Geometry: final body of the model. Coordinates: model frame, mm. Give positions to 0.01 mm unless a question says otherwise; leave off trailing zeros. Loops run counter-clockwise (first coordinate to the right, second up) from the corner with the lowest first, then second, coordinate; pieces in that order, holes last.
```python
from build123d import *

# Parameters (mm, degrees)
SKETCH5_R           = 48.26
BOSS_EXTRUDE1_DEPTH = 8.89
FILLET1_R           = 25.4
SKETCH9_R           = 2.5527
CUT_EXTRUDE1_DEPTH  = 12.7
FILLET3_R           = 12.7
FILLET4_R           = 12.7
FILLET5_R           = 5.08


with BuildPart() as part:
    # Sketch5 → Boss-Extrude1 (new body)
    with BuildSketch(Plane(origin=(0, 0, 0), x_dir=(1, 0, 0), z_dir=(0, 1, 0))):
        with BuildLine():
            ThreePointArc((-215.9, -46.097790831), (-267.470384182, -127.877406649), (-171.45, -139.168815315))
            Line((-171.45, -139.168815315), (-171.45, -167.709773326))
            Line((-171.45, -167.709773326), (-200.949318136, -200.960227902))
            Line((-200.949318136, -200.960227902), (-177.198993439, -222.031169428))
            Line((-177.198993439, -222.031169428), (-149.225, -190.5))
            Line((-149.225, -190.5), (-127, -190.5))
            Line((-127, -190.5), (-127, 190.5))
            Line((-127, 190.5), (-149.225, 190.5))
            Line((-149.225, 190.5), (-177.198993439, 222.031169428))
            Line((-177.198993439, 222.031169428), (-200.949318136, 200.960227902))
            Line((-200.949318136, 200.960227902), (-171.45, 167.709773326))
            Line((-171.45, 167.709773326), (-171.45, 123.173233653))
            ThreePointArc((-171.45, 123.173233653), (-267.470384182, 111.881824988), (-215.9, 30.102209169))
            Line((-215.9, 30.102209169), (-215.9, -46.097790831))
        make_face()
        with Locations(Location((-215.9, -103.247790831, 0), (0, 0, 270))):
            Circle(SKETCH5_R, mode=Mode.SUBTRACT)
        with Locations(Location((-215.9, 87.252209169, 0), (0, 0, 270))):
            Circle(SKETCH5_R, mode=Mode.SUBTRACT)
    extrude(amount=-BOSS_EXTRUDE1_DEPTH)

    # Fillet1
    # the kernel refuses this fillet: 25.4 mm, written as the material it adds along each edge
    with BuildSketch(Plane(origin=(-171.45, 0, -123.173233653), x_dir=(0, 0, -1), z_dir=(0, -1, 0))) as fillet1_piece_1:
        with BuildLine():
            CenterArc((44.400828084, -25.4), FILLET1_R, 90, 103.342363797)
            Line((19.686411909, -31.261538462), (19.192123586, -31.378769231))
            ThreePointArc((19.192123586, -31.378769231), (12.009069237, -14.266854375), (-0.319297995, -0.395111111))
            Line((-0.319297995, -0.395111111), (0, 0.508))
            Line((0, 0.508), (44.400828084, 0.508))
            Line((44.400828084, 0.508), (44.400828084, 0))
        make_face()
    extrude(amount=8.89)
    with BuildSketch(Plane(origin=(-171.45, 0, 139.168815315), x_dir=(-0.8303696180979097, 0, 0.557212973054228), z_dir=(0, -1, 0))) as fillet1_piece_2:
        with BuildLine():
            CenterArc((41.297101209, -24.264819571), FILLET1_R, 107.194284187, 71.530497093)
            Line((15.903392067, -23.699544404), (15.395517884, -23.6882389))
            ThreePointArc((15.395517884, -23.6882389), (7.529868268, -12.132836392), (-0.421827766, -0.28306419))
            Line((-0.421827766, -0.28306419), (0.150171277, 0.485296391))
            ThreePointArc((0.150171277, 0.485296391), (16.894268676, -2.046155965), (33.638366076, 0.485296391))
            Line((33.638366076, 0.485296391), (33.788537353, 0))
        make_face()
    extrude(amount=8.89)

    # Sketch9 → Cut-Extrude1 (cut)
    with BuildSketch(Plane(origin=(0, 0, 0), x_dir=(1, 0, 0), z_dir=(0, 1, 0))):
        Polygon((-181.61, 8.105163913), (-181.61, 22.76986075), (-194.31, 30.102209169), (-207.01, 22.76986075), (-207.01, 8.105163913), (-194.31, 0.772815494), align=None)
        Polygon((-175.26, -46.887449227), (-175.26, -32.22275239), (-187.96, -24.890403971), (-200.66, -32.22275239), (-200.66, -46.887449227), (-187.96, -54.219797646), align=None)
        Polygon((-175.26, -24.890403971), (-162.56, -17.558055552), (-162.56, -2.893358715), (-175.26, 4.438989704), (-187.96, -2.893358715), (-187.96, -17.558055552), align=None)
        Polygon((-194.31, -6.559532924), (-203.345054514, -1.343141768), (-203.345054514, -26.440620918), (-194.31, -21.224229762), align=None)
        Polygon((-162.56, 33.768383379), (-162.56, 4.438989704), (-175.26, 11.771338122), (-175.26, 26.43603496), align=None)
        Polygon((-162.56, -24.890403971), (-162.56, -46.887449227), (-168.91, -43.221275018), (-168.91, -28.55657818), align=None)
        with Locations(Location((-183.436118723, -153.432579675, 0), (0, 0, 270))):
            Circle(SKETCH9_R)
        with Locations(Location((-138.1125, 183.418546383, 0), (0, 0, 270))):
            Circle(SKETCH9_R)
        with Locations(Location((-138.1125, -184.15, 0), (0, 0, 270))):
            Circle(SKETCH9_R)
        with Locations(Location((-166.939936911, 153.157179019, 0), (0, 0, 270))):
            Circle(SKETCH9_R)
        with Locations(Location((-209.55, -1.647790831, 0), (0, 0, 270))):
            Circle(SKETCH9_R)
        with Locations(Location((-209.55, -33.397790831, 0), (0, 0, 270))):
            Circle(SKETCH9_R)
        with Locations(Location((-209.55, 30.102209169, 0), (0, 0, 270))):
            Circle(SKETCH9_R)
    extrude(amount=-CUT_EXTRUDE1_DEPTH, mode=Mode.SUBTRACT)

    # Fillet3
    fillet3_edges = [part.edges().sort_by_distance(p)[0] for p in [
        (-149.225, -4.445, -190.5),
        (-171.45, -4.445, -167.709773326),
        (-171.45, -4.445, 167.709773326),
        (-149.225, -4.445, 190.5),
    ]]
    fillet(fillet3_edges, radius=FILLET3_R)

    # Fillet4
    fillet4_edges = [part.edges().sort_by_distance(p)[0] for p in [
        (-215.9, -4.445, 46.097790831),
        (-215.9, -4.445, -30.102209169),
    ]]
    fillet(fillet4_edges, radius=FILLET4_R)

    # Fillet5
    fillet5_edges = [part.edges().sort_by_distance(p)[0] for p in [
        (-200.949318136, -4.445, -200.960227902),
        (-177.198993439, -4.445, -222.031169428),
    ]]
    fillet(fillet5_edges, radius=FILLET5_R)


solid = part.part
```
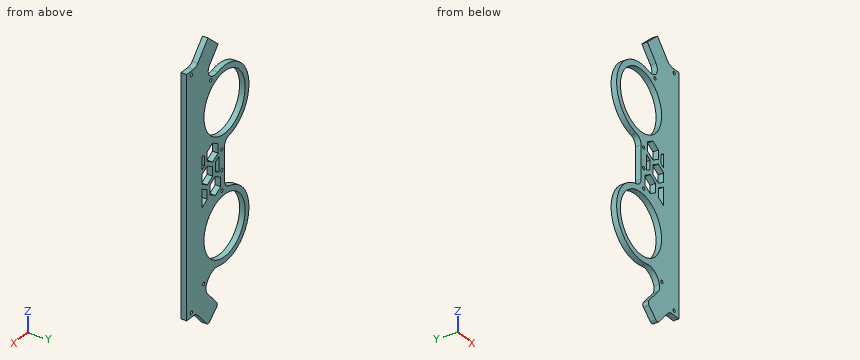
Q1. Pin query (flat end, axial travel): pin 1 Ø4 at (x, z) = (-209.55, 33.4) entering from +Y; pin 2 Ø2.5 at (y, z) = (-6, 38.5) entering from -X; pin 3 Ø2.5 at (x, y) = (-133, -6) entering from +Z; pin 4 Ø4.5 at (y, z) = (-5, -17) entering from -X. Return the tip coordinate at first contact, or that it passes through.
Q2. Material intervals for probe 1 along Z at (x, y) = (-137, -8.5); probe 2 along Z at (x, y) = (-222, -2); probe 3 along X at (y, z) = (-7, 184.15), sorted ascending.
Q3. Section query C-C, the plane z = -50.5. Return loops of the section in (x, y).
Q4. Section query B-B, the plane y = -5.25. State how many separate pieces and enclosed holes the cut face has, and give its area (3 significant figures).
Q5. Section query A-A, the plane z = 109. Return loops of the section in (x, y).
Resolved:
1. pin 1: passes through
1. pin 2: stops at x = -217.01
1. pin 3: stops at z = 190.5
1. pin 4: stops at x = -215.92
2. probe 1: z = -190.5 to -185.72, -181.12 to 181.85, 186.45 to 190.5
2. probe 2: z = -144.08 to -135.13, -39.38 to -29.42, 45.41 to 55.37, 151.12 to 160.07
2. probe 3: x = -186.04 to -140.67, -135.56 to -127
3. outline: (-259.67, -8.89) - (-247.18, -8.89) - (-247.18, 0) - (-259.67, 0) - close; (-184.62, -8.89) - (-127, -8.89) - (-127, 0) - (-184.62, 0) - close
4. separate pieces: 1
4. enclosed holes: 15
4. area: 26,100 mm2
5. outline: (-272.76, -8.89) - (-263.82, -8.89) - (-263.82, 0) - (-272.76, 0) - close; (-167.98, -8.89) - (-127, -8.89) - (-127, 0) - (-167.98, 0) - close
